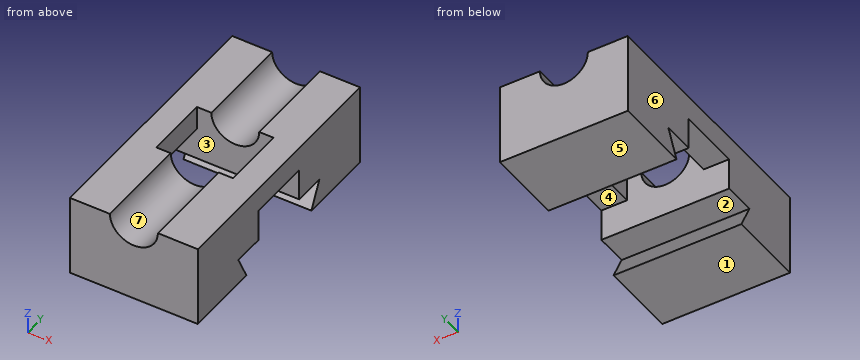
from build123d import *

# Parameters (mm, degrees)
BOSS_EXTRUDE1_DEPTH     = 10
CUT_EXTRUDE2_DEPTH      = 4.88
CUT_EXTRUDE4_DEPTH      = 18.67766953
CUT_EXTRUDE4_DEPTH_BACK = 18.67766953
SKETCH6_3_R             = 1.875
CUT_EXTRUDE5_DEPTH      = 24.58495283
CUT_EXTRUDE5_DEPTH_BACK = 24.58495283
SKETCH7_OUTSIDE_W       = 17.386
SKETCH7_OUTSIDE_H       = 22.386
SKETCH7_OUTSIDE_W_2     = 10
SKETCH7_OUTSIDE_H_2     = 6.38


with BuildPart() as part:
    # Sketch2 → Boss-Extrude1 (new body)
    with BuildSketch(Plane.YZ):
        Polygon((-10, -7.5), (-4, -7.5), (-5, -5.5), (-2.5, -5.5), (-2.5, -3), (2.5, -3), (2.5, -5.5), (5, -5.5), (4, -7.5), (10, -7.5), (10, 7.5), (-10, 7.5), align=None)
    extrude(amount=BOSS_EXTRUDE1_DEPTH)

    # Sketch4 → Cut-Extrude2 (cut)
    with BuildSketch(Plane(origin=(0, 0, -3), x_dir=(1, 0, 0), z_dir=(0, 0, -1))):
        Polygon((5, 2.5), (2, 2.5), (2, -2.5), (8, -2.5), (8, 2.5), align=None)
    extrude(amount=-CUT_EXTRUDE2_DEPTH, mode=Mode.SUBTRACT)

    # Sketch6_3 → Cut-Extrude4 (cut, two sides: drawn at the far end of the back side and taken through both)
    with BuildSketch(Plane.XZ.offset(-2.5).offset(-CUT_EXTRUDE4_DEPTH_BACK)):
        with Locations(Location((5, -1.12, 0), (0, 0, 270))):
            Circle(SKETCH6_3_R)
    extrude(amount=CUT_EXTRUDE4_DEPTH + CUT_EXTRUDE4_DEPTH_BACK, mode=Mode.SUBTRACT)

    # Sketch7 outside → Cut-Extrude5 (cut, two sides: drawn at the far end of the back side and taken through both)
    with BuildSketch(Plane(origin=(0, 10, 0), x_dir=(-1, 0, 0), z_dir=(0, 1, 0)).offset(-CUT_EXTRUDE5_DEPTH_BACK)):
        with Locations((-5, 0)):
            Rectangle(SKETCH7_OUTSIDE_W, SKETCH7_OUTSIDE_H)
        with Locations((-5, -4.31)):
            Rectangle(SKETCH7_OUTSIDE_W_2, SKETCH7_OUTSIDE_H_2, mode=Mode.SUBTRACT)
    extrude(amount=CUT_EXTRUDE5_DEPTH + CUT_EXTRUDE5_DEPTH_BACK, mode=Mode.SUBTRACT)


solid = part.part
Check sheet for the modelled part. Datum: model origin and axes. Units: mm. Face numbers are marked on the shaded views. A direction names the side the tool comes from. Round coordinates to 2 decimals unless told otherwise and drop trailing zeros. Write each loop counter-clockwise with the first axis right and the second up, starting at its lowest first coordinate (ties: lowest second). Pieces come first, ordered by that corner, then holes. Notation, with made-up numbers: (7, 15.5) - (30, 15.5) arc R15 cw to (30, 35.5) - close; hole circle Ø10 at (34, 88). An arc over 180 degrees is marked (long way). Return JSON: item names as keys, results as strings.
Q1. Depth check by flat-ended pin: P1, Ø2, axis at x = 8, y = 2.5, coming from the -Z side; P2, Ø3, axis at x = 3, y = 3.5, coming from the -Z side; P3, Ø1, axis at x = 5.5, y = 6, coming from the +Z side; P4, Ø1.6, axis at x = 1.5, y = 1, coming from the -Z side. Enter the tip coordinate at first touch or a pass-through.
Returned:
{"P1": "stops at z = -5.5", "P2": "stops at z = -7.5", "P3": "stops at z = -2.71", "P4": "stops at z = -3"}
Q2. Scan lines: L1, parallel to Y at x = 2.25, z = -4.75; L2, parallel to X at y = -8, z = -1.25; L3, parallel to Z at x = 8.25, y = 1.5. Record each from-to range of solid material in increasing order. Write a range as from..to.
Returned:
{"L1": "y = -10..-2.5, 2.5..10", "L2": "x = 0..3.13, 6.87..10", "L3": "z = -3..-1.12"}
Q3. Draft check along X on the marked faces 5, 6 and 7. Enter one of: released by +X, released by -X, zero draft, split by the parting line, or undercut.
Returned:
{"face 5": "zero draft", "face 6": "released by -X", "face 7": "undercut"}
Q4. Cross-section at A-A (y = -4.5). Record the boundary of the cut face in (x, z) (3 decimals), then the cut area to 3 significant figures.
Returned:
{"outline": "(0, -7.5) - (10, -7.5) - (10, -6.5) - (0, -6.5) - close; (0, -5.5) - (10, -5.5) - (10, -1.12) - (6.875, -1.12) arc R1.875 cw to (3.125, -1.12) - (0, -1.12) - close", "area": "48.3 mm²"}
Q5. Access from +Z, -Z, +X, -X, +Y, -Y to the whole of each face (thin tool, end or side, straight path). Record for the marked faces 1, 2, 3 and 4.
Returned:
{"face 1": "-Z, +X, -X, +Y, -Y", "face 2": "+X, -X", "face 3": "-Z", "face 4": "-Z, +X, -X"}
Q6. Cross-section at C-C (z = -4.5). Record the boundary of the cut face in (x, y).
Returned:
{"outline": "(0, -10) - (10, -10) - (10, -2.5) - (0, -2.5) - close; (0, 2.5) - (10, 2.5) - (10, 10) - (0, 10) - close"}
Q7. Cross-section at B-B (x = 2.25). Record the boundary of the cut face in (y, z), then the cut area to 3 significant figures.
Returned:
{"outline": "(-10, -7.5) - (-4, -7.5) - (-5, -5.5) - (-2.5, -5.5) - (-2.5, -1.12) - (-10, -1.12) - close; (2.5, -5.5) - (5, -5.5) - (4, -7.5) - (10, -7.5) - (10, -1.12) - (2.5, -1.12) - close", "area": "87.7 mm²"}
Q8. Cross-section at D-D (x = 5). Record the boundary of the cut face in (y, z) (3 decimals), then the cut area to 3 significant figures.
Returned:
{"outline": "(-10, -7.5) - (-4, -7.5) - (-5, -5.5) - (-2.5, -5.5) - (-2.5, -2.995) - (-10, -2.995) - close; (2.5, -5.5) - (5, -5.5) - (4, -7.5) - (10, -7.5) - (10, -2.995) - (2.5, -2.995) - close", "area": "59.6 mm²"}
